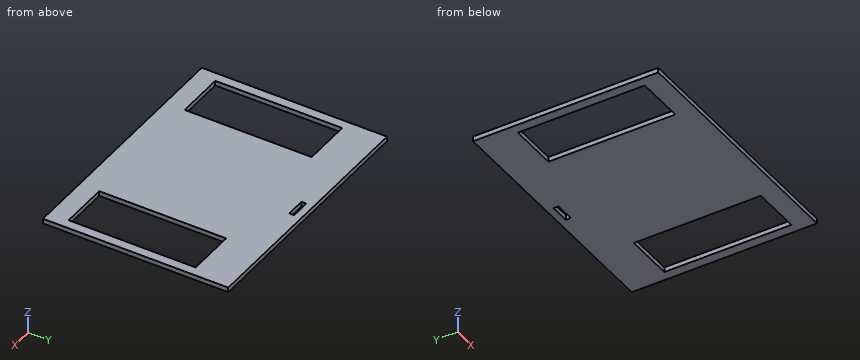
from build123d import *

# Parameters (mm, degrees)
F0_W     = 12.7
F0_H     = 3.175
F1_DEPTH = 3.175


# Not quite as in the source:
# - a feature names something its author has since deleted; it is built from what else it names


with BuildPart() as f1:
    # F0 (on Top) → F1 (new body)
    with BuildSketch(Plane.XY):
        Polygon((0, -12.7), (0, -120.396), (6.35, -120.396), (6.35, -37.846), (38.1, -37.846), (38.1, -120.396), (127, -120.396), (127, -37.846), (158.75, -37.846), (158.75, -120.396), (165.1, -120.396), (165.1, -12.7), align=None)
        with Locations((82.55, -19.05)):
            Rectangle(F0_W, F0_H, mode=Mode.SUBTRACT)
        Polygon((6.35, -120.396), (0, -120.396), (0, -133.096), (165.1, -133.096), (165.1, -120.396), (158.75, -120.396), (127, -120.396), (38.1, -120.396), align=None)
    extrude(amount=F1_DEPTH)


solid = f1.part
CAD build for the part. Positions are in the model's coordinates, mm. Round coordinates to 2 decimals unless told otherwise and drop trailing zeros. Write each loop counter-clockwise with the first axis right and the second up, starting at its lowest first coordinate (ties: lowest second). Pieces come first, ordered by that corner, then holes.
(1) Slice it at D-D, the plane x = 23. Write the cut outline in (y, z) (3 decimals).
(2) Slice it at A-A, the plane y = -64. Write the cut outline in (x, z) (3 decimals), and give its area (3 significant figures).
(3) Slice it at B-B, the plane x = 84.5. Write the cut outline in (y, z) (1 decimal).
(4) Probe line 1 along X through (y, z) = (-103.5, 0.3); line 2 along Y through (x, z) = (135.5, 1.45). List the from-to ranges inside material, lowest first.
(5) Slice it at C-C, the plane z = 0.75. Write the cut outline in (x, y), and give its area (3 significant figures).
From the geometry:
1. outline: (-133.096, 0) - (-120.396, 0) - (-120.396, 3.175) - (-133.096, 3.175) - close; (-37.846, 0) - (-12.7, 0) - (-12.7, 3.175) - (-37.846, 3.175) - close
2. outline: (0, 0) - (6.35, 0) - (6.35, 3.175) - (0, 3.175) - close; (38.1, 0) - (127, 0) - (127, 3.175) - (38.1, 3.175) - close; (158.75, 0) - (165.1, 0) - (165.1, 3.175) - (158.75, 3.175) - close
2. area: 323 mm2
3. outline: (-133.1, 0) - (-20.6, 0) - (-20.6, 3.2) - (-133.1, 3.2) - close; (-17.5, 0) - (-12.7, 0) - (-12.7, 3.2) - (-17.5, 3.2) - close
4. line 1: x = 0 to 6.35, 38.1 to 127, 158.75 to 165.1
4. line 2: y = -133.1 to -120.4, -37.85 to -12.7
5. outline: (0, -133.1) - (165.1, -133.1) - (165.1, -12.7) - (0, -12.7) - close; hole (6.35, -120.4) - (38.1, -120.4) - (38.1, -37.85) - (6.35, -37.85) - close; hole (76.2, -20.64) - (88.9, -20.64) - (88.9, -17.46) - (76.2, -17.46) - close; hole (127, -120.4) - (158.75, -120.4) - (158.75, -37.85) - (127, -37.85) - close
5. area: 14,600 mm2
